Verification items for the finished model (mm, model axes). A direction names the side the tool comes from. Round coordinates to 2 decimals unless told otherwise and drop trailing zeros. Order: outer loops, then holes, each group sorted by start corner. A loop starts at its lowest first (then second) coordinate and runs counter-clockwise, first axis right, second up. Notation, with made-up numbers: M 11,22 L 32,22 A5 ccw 32,27 Z; hole C 50.25,-26 d7. An arc over 180 degrees is marked long. Use CSV: the item, a comma, the result in double quotes. Start each with the question number.
Q1. Scan lines: line 1 (X direction, y = 17, z = 1.5); line 2 (Y direction, x = 41.5, z = 1.25); line 3 (Y direction, x = 24, z = 2.75). Record each from-to range of solid material in increasing order.
Q2. Sectioned sample at C-C (z = 7.5). Enter the section's corners in (x, y), and give its area (3 significant figures).
Q3. Gauge pin test, flat ends, axial feed: pin 1 Ø3 at (x, y) = (5.5, 7) entering from +Z; pin 2 Ø1 at (y, z) = (14.5, 3) entering from +X; pin 3 Ø1.6 at (x, y) = (0.5, 12) entering from +Z. Record the tip position at first contact, or that the pin passes through.
Q4. Sectioned sample at B-B (x = 42). Enter the section's corners in (y, z), and give its area (3 significant figures).
Q5. Sectioned sample at A-A (z = 2.5). Enter the section's corners in (x, y).
Q6. Mould release check, pull along Y, two halves, no side actions. Record for faces 5 (the face through (0, 14, 4)), 6 (the face through (26, 28.5, 5)), 7 (the face through (38, 14, 4)), 8 (the face through (26, 0, 5)): +Y half, -Y half, draft (parallel to the pull), parting line (faces both ways), or undercut.
Q7. Set-up check for faces 1 (the face through (16, 14, 4)), 2 (the face through (8, 14, 2)), 3 (the face through (1, 9.25, 7)), 4 (the face through (22, 27, 10)): record each of +Z, -Z, +X, -X, +Y, -Y from which the full face is reachable in a straight line by a thin tool's end or side.
Q8. Sectioned sample at D-D (y = 13.25). Enter the section's corners in (x, z).
```python
from build123d import *

# Parameters (mm, degrees)
F0_W     = 5
F0_H     = 16.5
F0_W_2   = 10
F0_H_2   = 8.5
F1_DEPTH = 1
F2_DEPTH = 4
F0_W_3   = 2
F0_H_3   = 10
F3_DEPTH = 5
F0_W_4   = 50
F0_H_4   = 2
F4_DEPTH = 10


# Not quite as in the source:
# - a feature names something its author has since deleted; it is built from what else it names


with BuildPart() as f1:
    # F0 (on Top) → F1 (new body)
    with BuildSketch(Plane.XY):
        Polygon((2, 6), (2, 2), (52, 2), (52, 6), (52, 26.5), (2, 26.5), (2, 22.5), (8, 22.5), (8, 6), align=None)
        with Locations((16.5, 14.25)):
            Rectangle(F0_W, F0_H, mode=Mode.SUBTRACT)
        with Locations((38.3, 14.25)):
            Rectangle(F0_W_2, F0_H_2, mode=Mode.SUBTRACT)
    extrude(amount=F1_DEPTH)

    # F0 (on Top) → F2 (join)
    with BuildSketch(Plane.XY):
        Polygon((2, 19.25), (2, 9.25), (2, 6), (8, 6), (8, 22.5), (2, 22.5), align=None)
        with Locations((16.5, 14.25)):
            Rectangle(F0_W, F0_H)
        with Locations((38.3, 14.25)):
            Rectangle(F0_W_2, F0_H_2)
    extrude(amount=F2_DEPTH)

    # F0 (on Top) → F3 (join)
    with BuildSketch(Plane.XY):
        with Locations((1, 14.25)):
            Rectangle(F0_W_3, F0_H_3)
    extrude(amount=F3_DEPTH)

    # F0 (on Top) → F4 (join)
    with BuildSketch(Plane.XY):
        with Locations((27, 27.5)):
            Rectangle(F0_W_4, F0_H_4)
        Polygon((0, 28.5), (0, 19.25), (2, 19.25), (2, 22.5), (2, 26.5), (2, 28.5), align=None)
        Polygon((0, 9.25), (0, 0), (2, 0), (2, 2), (2, 6), (2, 9.25), align=None)
        with Locations((27, 1)):
            Rectangle(F0_W_4, F0_H_4)
    extrude(amount=F4_DEPTH)


solid = f1.part
```
Verdict:
1,line 1,"x = 0 to 8, 14 to 19, 33.3 to 43.3"
1,line 2,"y = 0 to 2, 10 to 18.5, 26.5 to 28.5"
1,line 3,"y = 0 to 2, 26.5 to 28.5"
2,outline,"M 0,0 L 52,0 L 52,2 L 2,2 L 2,9.25 L 0,9.25 Z; M 0,19.25 L 2,19.25 L 2,26.5 L 52,26.5 L 52,28.5 L 0,28.5 Z"
2,area,"237 mm²"
3,pin 1,"stops at z = 4"
3,pin 2,"stops at x = 43.3"
3,pin 3,"stops at z = 5"
4,outline,"M 0,0 L 28.5,0 L 28.5,10 L 26.5,10 L 26.5,1 L 18.5,1 L 18.5,4 L 10,4 L 10,1 L 2,1 L 2,10 L 0,10 Z"
4,area,"90.0 mm²"
5,outline,"M 0,0 L 52,0 L 52,2 L 2,2 L 2,6 L 8,6 L 8,22.5 L 2,22.5 L 2,26.5 L 52,26.5 L 52,28.5 L 0,28.5 Z; M 14,6 L 19,6 L 19,22.5 L 14,22.5 Z; M 33.3,10 L 43.3,10 L 43.3,18.5 L 33.3,18.5 Z"
6,face 5,"draft"
6,face 6,"+Y half"
6,face 7,"undercut"
6,face 8,"-Y half"
7,face 1,"+Z, +X"
7,face 2,"+Z"
7,face 3,"+Z, +X, -X"
7,face 4,"+Z, +X, -X, +Y, -Y"
8,outline,"M 0,0 L 52,0 L 52,1 L 43.3,1 L 43.3,4 L 33.3,4 L 33.3,1 L 19,1 L 19,4 L 14,4 L 14,1 L 8,1 L 8,4 L 2,4 L 2,5 L 0,5 Z"
